from build123d import *

# Parameters (mm, degrees)
BASE_FLANGE1_DEPTH  = 19
CUT_EXTRUDE1_DEPTH  = 0.33
TAB1_DEPTH          = 0.33
CUT_EXTRUDE2_DEPTH  = 21.457693541
SKETCH_1_W          = 4.170383739
SKETCH_1_H          = 15.60949608
CUT_EXTRUDE_1_DEPTH = 1.6


# Sheet-metal steps are written as plain solids
with BuildPart() as part:
    # Sketch1 → Base-Flange1 (new body)
    with BuildSketch(Plane(origin=(0, 0, 0), x_dir=(0, 0, -1), z_dir=(1, 0, 0))):
        with BuildLine():
            Line((0.01, 2.27), (5.595, 2.27))
            ThreePointArc((5.595, 2.27), (5.934411255, 2.129411255), (6.075, 1.79))
            Line((6.075, 1.79), (6.075, -1.79))
            ThreePointArc((6.075, -1.79), (5.934411255, -2.129411255), (5.595, -2.27))
            Line((5.595, -2.27), (-5.595, -2.27))
            ThreePointArc((-5.595, -2.27), (-5.934411255, -2.129411255), (-6.075, -1.79))
            Line((-6.075, -1.79), (-6.075, 1.79))
            ThreePointArc((-6.075, 1.79), (-5.934411255, 2.129411255), (-5.595, 2.27))
            Line((-5.595, 2.27), (-0.01, 2.27))
            Line((-0.01, 2.27), (-0.01, 1.94))
            Line((-0.01, 1.94), (-5.595, 1.94))
            ThreePointArc((-5.595, 1.94), (-5.701066017, 1.896066017), (-5.745, 1.79))
            Line((-5.745, 1.79), (-5.745, -1.79))
            ThreePointArc((-5.745, -1.79), (-5.701066017, -1.896066017), (-5.595, -1.94))
            Line((-5.595, -1.94), (5.595, -1.94))
            ThreePointArc((5.595, -1.94), (5.701066017, -1.896066017), (5.745, -1.79))
            Line((5.745, -1.79), (5.745, 1.79))
            ThreePointArc((5.745, 1.79), (5.701066017, 1.896066017), (5.595, 1.94))
            Line((5.595, 1.94), (0.01, 1.94))
            Line((0.01, 1.94), (0.01, 2.27))
        make_face()
    extrude(amount=BASE_FLANGE1_DEPTH)

    # Sketch6 → Cut-Extrude1 (cut)
    with BuildSketch(Plane(origin=(0, 2.27, 0), x_dir=(1, 0, 0), z_dir=(0, 1, 0))):
        with BuildLine():
            Line((16.5, 0.01), (16.5, -1.15))
            ThreePointArc((16.5, -1.15), (16.470710678, -1.220710678), (16.4, -1.25))
            Line((16.4, -1.25), (15.24, -1.25))
            ThreePointArc((15.24, -1.25), (15.169289322, -1.220710678), (15.14, -1.15))
            Line((15.14, -1.15), (15.14, 0.01))
            Line((15.14, 0.01), (16.5, 0.01))
        make_face()
        with BuildLine():
            Line((3.86, 0.01), (2.5, 0.01))
            Line((2.5, 0.01), (2.5, -1.15))
            ThreePointArc((2.5, -1.15), (2.529289322, -1.220710678), (2.6, -1.25))
            Line((2.6, -1.25), (3.76, -1.25))
            ThreePointArc((3.76, -1.25), (3.830710678, -1.220710678), (3.86, -1.15))
            Line((3.86, -1.15), (3.86, 0.01))
        make_face()
    extrude(amount=-CUT_EXTRUDE1_DEPTH, mode=Mode.SUBTRACT)

    # Sketch7 → Tab1 (add)
    with BuildSketch(Plane(origin=(0, 2.27, 0), x_dir=(1, 0, 0), z_dir=(0, 1, 0))):
        with BuildLine():
            Line((15.16, -0.01), (15.16, 0.01))
            Line((15.16, 0.01), (16.48, 0.01))
            Line((16.48, 0.01), (16.48, -0.01))
            Line((16.48, -0.01), (16.48, -1.15))
            ThreePointArc((16.48, -1.15), (16.456568542, -1.206568542), (16.4, -1.23))
            Line((16.4, -1.23), (15.24, -1.23))
            ThreePointArc((15.24, -1.23), (15.183431458, -1.206568542), (15.16, -1.15))
            Line((15.16, -1.15), (15.16, -0.01))
        make_face()
        with BuildLine():
            Line((2.52, -0.01), (2.52, 0.01))
            Line((2.52, 0.01), (3.84, 0.01))
            Line((3.84, 0.01), (3.84, -0.01))
            Line((3.84, -0.01), (3.84, -1.15))
            ThreePointArc((3.84, -1.15), (3.816568542, -1.206568542), (3.76, -1.23))
            Line((3.76, -1.23), (2.6, -1.23))
            ThreePointArc((2.6, -1.23), (2.543431458, -1.206568542), (2.52, -1.15))
            Line((2.52, -1.15), (2.52, -0.01))
        make_face()
    extrude(amount=-TAB1_DEPTH)

    # Sketch10 → Cut-Extrude2 (cut, through all)
    with BuildSketch(Plane(origin=(0, 2.27, 0), x_dir=(1, 0, 0), z_dir=(0, 1, 0))):
        with BuildLine():
            Line((11.9, -1.84), (13.65, -1.84))
            ThreePointArc((13.65, -1.84), (13.720710678, -1.869289322), (13.75, -1.94))
            Line((13.75, -1.94), (13.75, -4.16))
            ThreePointArc((13.75, -4.16), (13.720710678, -4.230710678), (13.65, -4.26))
            Line((13.65, -4.26), (11.9, -4.26))
            ThreePointArc((11.9, -4.26), (11.829289322, -4.230710678), (11.8, -4.16))
            Line((11.8, -4.16), (11.8, -1.94))
            ThreePointArc((11.8, -1.94), (11.829289322, -1.869289322), (11.9, -1.84))
        make_face()
        with BuildLine():
            Line((13.75, 1.96), (13.75, 4.18))
            ThreePointArc((13.75, 4.18), (13.720710678, 4.250710678), (13.65, 4.28))
            Line((13.65, 4.28), (11.9, 4.28))
            ThreePointArc((11.9, 4.28), (11.829289322, 4.250710678), (11.8, 4.18))
            Line((11.8, 4.18), (11.8, 1.96))
            ThreePointArc((11.8, 1.96), (11.829289322, 1.889289322), (11.9, 1.86))
            Line((11.9, 1.86), (13.65, 1.86))
            ThreePointArc((13.65, 1.86), (13.720710678, 1.889289322), (13.75, 1.96))
        make_face()
    extrude(amount=-CUT_EXTRUDE2_DEPTH, mode=Mode.SUBTRACT)

    # Эскиз1 → Вырез-Вытянуть1 (cut)
    with BuildSketch(Plane(origin=(0, 2.27, 0), x_dir=(1, 0, 0), z_dir=(0, 1, 0))):
        with Locations((1.41480813, -0.01)):
            Rectangle(SKETCH_1_W, SKETCH_1_H)
    extrude(amount=-CUT_EXTRUDE_1_DEPTH, mode=Mode.SUBTRACT)


solid = part.part
Part model, mm, in its own coordinate system. A direction names the side the tool comes from. Round coordinates to 2 decimals unless told otherwise and drop trailing zeros. Write each loop counter-clockwise with the first axis right and the second up, starting at its lowest first coordinate (ties: lowest second). Pieces come first, ordered by that corner, then holes. Notation, with made-up numbers: M -22.75,25 L 9.25,25 A26 cw 9.25,51 Z; hole C 46,20 d7. An arc over 180 degrees is marked long. Return JSON: item names as keys, results as strings. Group by question number.
(1) Pin check, flat tip, straight feed: pin 1 Ø0.5 at (y, z) = (2, 3.5) entering from -X. Stop position of the tip, or through.
(2) Two-plate mould, pull along Z, no slides. Class faces 1 (the face through (9, 0, -5.745)), 2 (the face through (9, 0, 6.075)), 3 (the face through (9, -1.94, 0)), 4 (the face through (3.5, 2.1, -2.7)): +Z half, -Z half, draft (parallel to the pull), parting line (faces both ways), or undercut.
(3) Saw through at A-A on y = -1.5. Write the cut outline in (x, z) (3 decimals), then the cut area to 3 significant figures.
(4) Saw through at D-D on z = -0.25. Write the cut outline in (x, y), then the cut area to 3 significant figures.
(5) Saw through at C-C on x = 17. Write the cut outline in (y, z) (3 decimals), then the cut area to 3 significant figures.
(6) Saw through at B-B on z = 2.75. Write the cut outline in (x, y).
(7) Which spindle directions (+Z, -Z, +X, -X, +Y, -Y) get a long thin tool onto all of the face, cutting with end or side? Do faces 5 (the face through (9, 0, 5.745)), 6 (the face through (11, 2.27, 3)), 7 (the face through (3.5, 2.1, 4)). Say none if no direction does.
(8) Drill centre lines: probe 1 along Y at (x, z) = (10.75, 1.5); probe 2 along Z at (x, y) = (8.5, 0.75) (3 decimals); probe 3 along Y at (x, z) = (1.25, 5.5). Where is each one in solid material? Low to high.
Returned:
{
 "1": {"pin 1": "x = 3.5"},
 "2": {"face 1": "undercut", "face 2": "+Z half", "face 3": "undercut", "face 4": "draft"},
 "3": {"outline": "M 0,-6.075 L 19,-6.075 L 19,-5.745 L 0,-5.745 Z; M 0,5.745 L 19,5.745 L 19,6.075 L 0,6.075 Z", "area": "12.5 mm²"},
 "4": {"outline": "M 0,-2.27 L 19,-2.27 L 19,-1.94 L 0,-1.94 Z; M 3.5,1.94 L 19,1.94 L 19,2.27 L 3.5,2.27 Z", "area": "11.4 mm²"},
 "5": {"outline": "M -2.27,-5.595 A0.48 ccw -1.79,-6.075 L 1.79,-6.075 A0.48 ccw 2.27,-5.595 L 2.27,-0.01 L 1.94,-0.01 L 1.94,-5.595 A0.15 cw 1.79,-5.745 L -1.79,-5.745 A0.15 cw -1.94,-5.595 L -1.94,5.595 A0.15 cw -1.79,5.745 L 1.79,5.745 A0.15 cw 1.94,5.595 L 1.94,0.01 L 2.27,0.01 L 2.27,5.595 A0.48 ccw 1.79,6.075 L -1.79,6.075 A0.48 ccw -2.27,5.595 Z", "area": "10.4 mm²"},
 "6": {"outline": "M 0,-2.27 L 11.8,-2.27 L 11.8,-1.94 L 0,-1.94 Z; M 3.5,1.94 L 11.8,1.94 L 11.8,2.27 L 3.5,2.27 Z; M 13.75,-2.27 L 19,-2.27 L 19,-1.94 L 13.75,-1.94 Z; M 13.75,1.94 L 19,1.94 L 19,2.27 L 13.75,2.27 Z"},
 "7": {"face 5": "+X, -X", "face 6": "+Z, -Z, +X, -X, +Y", "face 7": "+Z, -Z, -X, +Y"},
 "8": {"probe 1": "-2.27 to -1.94, 1.94 to 2.27", "probe 2": "-6.075 to -5.745, 5.745 to 6.075", "probe 3": "-2.27 to -1.94"}
}
